Build history of the part. All positions in model axes, mm. A direction names the side the tool comes from. Give positions to 0.01 mm unless a question says otherwise; leave off trailing zeros. Loops run counter-clockwise (first coordinate to the right, second up) from the corner with the lowest first, then second, coordinate; pieces in that order, holes last. Notation, with made-up numbers: (-32.75, 23.5) -> (-0.75, 23.5) arc R16 cw to (-0.75, 42.5) -> close; hole circle Ø5 at (13.5, -13.75). An arc over 180 degrees is marked (long way). Answer in a Markdown table with one row per item. Add a question column.
from build123d import *

# Parameters (mm, degrees)
SKETCH1_W                = 50
SKETCH1_H                = 4
BOSS_EXTRUDE1_DEPTH      = 7
M4_CLEARANCE_HOLE1_D     = 4.5
CUT_EXTRUDE1_DEPTH       = 78.259303647
CUT_EXTRUDE1_DEPTH_BACK  = 78.259303647
CUT_EXTRUDE2_DEPTH       = 2.8
M3_CLEARANCE_HOLE1_D     = 3.4
M3_CLEARANCE_HOLE1_DEPTH = 16
M3_CLEARANCE_HOLE1_TIP   = 1.021463052
FILLET1_R                = 3


with BuildPart() as part:
    # Sketch1 → Boss-Extrude1 (new, symmetric)
    with BuildSketch(Plane(origin=(0, 0, 0), x_dir=(1, 0, 0), z_dir=(0, 1, 0))):
        Polygon((50, 4), (50, 0), (56, 0), (56, 4.5), (76, 4.5), (76, 8), (50, 8), align=None)
        Polygon((50, 0), (50, -4), (50, -8), (76, -8), (76, -4.5), (56, -4.5), (56, 0), align=None)
        with Locations((25, 2)):
            Rectangle(SKETCH1_W, SKETCH1_H)
        with Locations((25, -2)):
            Rectangle(SKETCH1_W, SKETCH1_H)
    extrude(amount=BOSS_EXTRUDE1_DEPTH, both=True)

    # M4 Clearance Hole1 (through all)
    with Locations(Plane(origin=(0, 0, -8), x_dir=(-1, 0, 0), z_dir=(0, 0, -1))):
        with Locations((-68, 0)):
            Hole(M4_CLEARANCE_HOLE1_D / 2)

    # Sketch6 → Cut-Extrude1 (cut, two sides: drawn at the far end of the back side and taken through both)
    with BuildSketch(Plane(origin=(0, 0, -4), x_dir=(-1, 0, 0), z_dir=(0, 0, -1)).offset(-CUT_EXTRUDE1_DEPTH_BACK)):
        with BuildLine():
            Line((-12, -2.5), (-22, -2.5))
            ThreePointArc((-22, -2.5), (-24.5, 0), (-22, 2.5))
            Line((-22, 2.5), (-12, 2.5))
            ThreePointArc((-12, 2.5), (-9.5, 0), (-12, -2.5))
        make_face()
    extrude(amount=CUT_EXTRUDE1_DEPTH + CUT_EXTRUDE1_DEPTH_BACK, mode=Mode.SUBTRACT)

    # Sketch7 → Cut-Extrude2 (cut)
    with BuildSketch(Plane.ZY.offset(-7)):
        Polygon((4, 2.9), (-1.924315781, 2.9), (-3.598631561, 0), (-1.924315781, -2.9), (4, -2.9), align=None)
    extrude(amount=CUT_EXTRUDE2_DEPTH, mode=Mode.SUBTRACT)

    # M3 Clearance Hole1
    with Locations(Plane(origin=(0, 0, 0), x_dir=(0, 0, -1), z_dir=(-1, 0, 0))):
        with Locations((0, 0)):
            Hole(M3_CLEARANCE_HOLE1_D / 2, depth=M3_CLEARANCE_HOLE1_DEPTH)
            with Locations((0, 0, -(M3_CLEARANCE_HOLE1_DEPTH + M3_CLEARANCE_HOLE1_TIP / 2))):  # 118° drill point
                Cone(0, M3_CLEARANCE_HOLE1_D / 2, M3_CLEARANCE_HOLE1_TIP, mode=Mode.SUBTRACT)

    # Fillet1
    fillet1_edges = [part.edges().sort_by_distance(p)[0] for p in [
        (0, 7, 0),
        (76, -7, -6.25),
        (76, -7, 6.25),
        (0, -7, 0),
        (50, 0, -8),
        (50, 0, 8),
        (76, 7, 6.25),
        (76, 7, -6.25),
    ]]
    fillet(fillet1_edges, radius=FILLET1_R)


solid = part.part
(1) 3-axis set-ups, long thin cutter, end or side, ignore diameter. For faces 4 (the cylindrical face through (10.12, 1.65, 0.94)), 5 (the cylindrical face through (2.13, 1.66, -0.37)), 6 (the flat face through (25, 0, 4)), 7 (the flat face through (56, 0, 0)), 8 (the flat face through (6, -2.9, 1)): which of +Z, -Z, +X, -X, +Y, -Y reach the whole face in a straight line?
(2) Saw through at D-D, the plane x = 39.5. List the corners of the cut face in (y, z).
(3) Saw through at B-B, the plane z = 0. List the corners of the cut face in (x, y), then the cut area to 3 significant figures.
(4) Wall check: line 1 along X through (y, z) = (-0.25, 1.75); line 2 along Y through (x, z) = (6.5, 1.5); line 3 along Y through (x, z) = (12.5, -1.75). Give the ranges that are in metal, low to high. Write a range as from..to.
(5) Two-plate mould, pull along X, no slides. Class faces 1 (the cylindrical face through (50.86, 0.1, 7.1)), 2 (the cylindrical face through (75.1, 6.14, 6.23)), 3 (the cylindrical face through (66.34, 1.52, 6.27)): released by +X, released by -X, zero draft, split by the parting line, or undercut.
(6) Saw through at A-A, the plane x = 68. List the corners of the cut face in (y, z).
(7) Flat gauge pins, fed straight in: pin 1 Ø2 at (y, z) = (0, 0) entering from -X; pin 2 Ø4 at (y, z) = (0, 0) entering from +X; pin 3 Ø0.5 at (y, z) = (0, -4.5) entering from -X; pin 4 Ø2.5 at (x, y) = (68, 0) entering from +Z. Where does each tip first touch, or does it go through?
(8) Saw through at C-C, the plane y = 5.25. List the corners of the cut face in (x, z), then the cut area to 3 significant figures.
Worked answers:
| question | item | result |
|---|---|---|
| 1 | face 4 | +Z, -Z |
| 1 | face 5 | -X |
| 1 | face 6 | +Z, -X, +Y, -Y |
| 1 | face 7 | +X, +Y, -Y |
| 1 | face 8 | +Z |
| 2 | outline | (-7, -4) -> (7, -4) -> (7, 4) -> (-7, 4) -> close |
| 3 | outline | (0, -4) arc R3 ccw to (3, -7) -> (56, -7) -> (56, 7) -> (3, 7) arc R3 ccw to (0, 4) -> (0, 1.7) -> (4.2, 1.7) -> (4.2, 2.9) -> (7, 2.9) -> (7, 1.7) -> (10.17, 1.7) arc R2.5 cw to (12, 2.5) -> (22, 2.5) arc R2.5 cw to (22, -2.5) -> (12, -2.5) arc R2.5 cw to (10.17, -1.7) -> (7, -1.7) -> (7, -2.9) -> (4.2, -2.9) -> (4.2, -1.7) -> (0, -1.7) -> close |
| 3 | area | 671 mm^2 |
| 4 | line 1 | 0..4.2, 7..9.51, 24.49..56 |
| 4 | line 2 | -7..-2.9, 2.9..7 |
| 4 | line 3 | -7..-2.5, 2.5..7 |
| 5 | face 1 | released by -X |
| 5 | face 2 | released by +X |
| 5 | face 3 | undercut |
| 6 | outline | (-7, -8) -> (-2.25, -8) -> (-2.25, -4.5) -> (-7, -4.5) -> close; (-7, 4.5) -> (-2.25, 4.5) -> (-2.25, 8) -> (-7, 8) -> close; (2.25, -8) -> (7, -8) -> (7, -4.5) -> (2.25, -4.5) -> close; (2.25, 4.5) -> (7, 4.5) -> (7, 8) -> (2.25, 8) -> close |
| 7 | pin 1 | x = 24.29 |
| 7 | pin 2 | x = 56 |
| 7 | pin 3 | x = 50 |
| 7 | pin 4 | through |
| 8 | outline | (0.27, -4) -> (50, -4) -> (50, -5) arc R3 ccw to (53, -8) -> (75.73, -8) -> (75.73, -4.5) -> (56, -4.5) -> (56, 4.5) -> (75.73, 4.5) -> (75.73, 8) -> (53, 8) arc R3 ccw to (50, 5) -> (50, 4) -> (0.27, 4) -> close |
| 8 | area | 628 mm^2 |
